```python
from build123d import *

# Parameters (mm, degrees)
SKETCH_1_R               = 4.1
EXTRUDE_1_DEPTH          = 10
SKETCH_2_W               = 10.2
SKETCH_2_H               = 10.2
CUT_EXTRUDE_1_DEPTH      = 5
SKETCH_3_W               = 10
SKETCH_3_H               = 10
EXTRUDE_2_DEPTH          = 10
CUT_EXTRUDE_2_DEPTH      = 64.876521508
CUT_EXTRUDE_2_DEPTH_BACK = 64.876521508
SKETCH_4_R               = 1.6


with BuildPart() as part:
    # ｽｹｯﾁ1 → ﾎﾞｽ - 押し出し1 (new body)
    with BuildSketch(Plane(origin=(0, 0, 0), x_dir=(1, 0, 0), z_dir=(0, 1, 0))):
        with BuildLine():
            Line((-47.110254718, 7.529627927), (-6.738797431, 34.929179684))
            ThreePointArc((-6.738797431, 34.929179684), (5.618470914, 35.603432679), (12, 25))
            Line((12, 25), (12, -25))
            ThreePointArc((12, -25), (5.618470914, -35.603432679), (-6.738797431, -34.929179684))
            Line((-6.738797431, -34.929179684), (-47.110254718, -7.529627927))
            ThreePointArc((-47.110254718, -7.529627927), (-51.1, 0), (-47.110254718, 7.529627927))
        make_face()
        with Locations(Location((-42, 0, 0), (0, 0, 270))):
            Circle(SKETCH_1_R, mode=Mode.SUBTRACT)
    extrude(amount=EXTRUDE_1_DEPTH)

    # ｽｹｯﾁ2 → ｶｯﾄ - 押し出し1 (cut)
    with BuildSketch(Plane.XZ):
        with Locations((0, 25)):
            Rectangle(SKETCH_2_W, SKETCH_2_H)
        with Locations((0, -25)):
            Rectangle(SKETCH_2_W, SKETCH_2_H)
        with Locations((-20, 0)):
            Rectangle(SKETCH_2_W, SKETCH_2_H)
    extrude(amount=-CUT_EXTRUDE_1_DEPTH, mode=Mode.SUBTRACT)

    # ｽｹｯﾁ3 → ﾎﾞｽ - 押し出し2 (add)
    with BuildSketch(Plane(origin=(12, 0, 0), x_dir=(0, 0, -1), z_dir=(1, 0, 0))):
        with Locations((-15, 5)):
            Rectangle(SKETCH_3_W, SKETCH_3_H)
        with Locations((15, 5)):
            Rectangle(SKETCH_3_W, SKETCH_3_H)
    extrude(amount=EXTRUDE_2_DEPTH)

    # ｽｹｯﾁ4 → ｶｯﾄ - 押し出し2 (cut, two sides: drawn at the far end of the back side and taken through both)
    with BuildSketch(Plane.XY.offset(-CUT_EXTRUDE_2_DEPTH_BACK)):
        with Locations((17, 5)):
            Circle(SKETCH_4_R)
    extrude(amount=CUT_EXTRUDE_2_DEPTH + CUT_EXTRUDE_2_DEPTH_BACK, mode=Mode.SUBTRACT)


solid = part.part
```
Input: part model. Units: mm. Frame: model coordinates. A direction names the side the tool comes from. Round coordinates to 2 decimals unless told otherwise and drop trailing zeros. Loops run counter-clockwise (first coordinate to the right, second up) from the corner with the lowest first, then second, coordinate; pieces in that order, holes last. Notation, with made-up numbers: (-22, 86.5) -> (0, 86.5) arc R9 cw to (0, 94.5) -> close; hole circle Ø3 at (-31.5, 46). An arc over 180 degrees is marked (long way). One line per item, written item: value.
(1) Section C-C (y = 1.75). Return the cut outline in (x, z).
Geometry check:
outline: (-47.11, -7.53) -> (-6.74, -34.93) arc R12 ccw to (12, -25) -> (12, -20) -> (22, -20) -> (22, -10) -> (12, -10) -> (12, 10) -> (22, 10) -> (22, 20) -> (12, 20) -> (12, 25) arc R12 ccw to (-6.74, 34.93) -> (-47.11, 7.53) arc R9.1 ccw to start; hole circle Ø8.2 at (-42, 0); hole (-25.1, -5.1) -> (-14.9, -5.1) -> (-14.9, 5.1) -> (-25.1, 5.1) -> close; hole (-5.1, -30.1) -> (5.1, -30.1) -> (5.1, -19.9) -> (-5.1, -19.9) -> close; hole (-5.1, 19.9) -> (5.1, 19.9) -> (5.1, 30.1) -> (-5.1, 30.1) -> close
(2) Set-up query: faces 5 (the face through (0, 5, 25)), 6 (the face through (15, 5, 10)), 7 (the face through (15, 5, 20)), 8 (the face through (22, 5, 15)). Return all of +Z, -Z, +X, -X, +Y, -Y with unobstructed straight access to the full face (end or side cutting, diameter ignored); none if empty.
Geometry check:
face 5: -Y
face 6: +X, +Y, -Y
face 7: +Z, +X, +Y, -Y
face 8: +Z, -Z, +X, +Y, -Y
(3) Material intervals for line 1 (Y direction, x = 17, z = -12.25); line 2 (Z direction, x = 17, y = 2.25); line 3 (X direction, y = 8, z = 0), sorted ascending. Write a range as [from, to].
Geometry check:
line 1: [0, 3.4], [6.6, 10]
line 2: [-20, -10], [10, 20]
line 3: [-51.1, -46.1], [-37.9, 12]
(4) Pin query (flat end, axial travel): pin 1 (2 mm diameter, centred on y = 5, z = 13, fed in from -X); pin 2 (3 mm diameter, centred on x = 17, y = 5, fed in from +Z); pin 3 (6 mm diameter, centred on x = 1, y = 1.5, fed in from -Z); pin 4 (4 mm diameter, centred on x = 17, y = 5, fed in from +Z). Return the tip coordinate at first contact, or that it passes through.
Geometry check:
pin 1: x = -40.52
pin 2: through
pin 3: z = -37
pin 4: z = 20
(5) Mould query, pull axis Z, two halves, no side actions, for faces 1 (the face through (-51.1, 4.9, 0.1)), 2 (the face through (-20, 2, -5.1)), 3 (the face through (5.779, 4.93, 35.517)), 4 (the face through (15.4, 5.07, 14.93)). Classes: pulls with the +Z half, pulls with the -Z half, needs draft (parallel to the pull), parting line crosses it, or undercut.
Geometry check:
face 1: parting line crosses it
face 2: undercut
face 3: pulls with the +Z half
face 4: needs draft
(6) Section A-A (z = 0). Return the cut outline in (x, y).
Geometry check:
outline: (-51.1, 0) -> (-46.1, 0) -> (-46.1, 10) -> (-51.1, 10) -> close; (-37.9, 0) -> (-25.1, 0) -> (-25.1, 5) -> (-14.9, 5) -> (-14.9, 0) -> (12, 0) -> (12, 10) -> (-37.9, 10) -> close
(7) Section D-D (x = -41). Return the cut outline in (y, z), plus the area to 3 significant figures.
Geometry check:
outline: (0, -11.68) -> (10, -11.68) -> (10, -3.98) -> (0, -3.98) -> close; (0, 3.98) -> (10, 3.98) -> (10, 11.68) -> (0, 11.68) -> close
area: 154 mm2
(8) Section B-B (x = 17). Return the cut outline in (y, z).
Geometry check:
outline: (0, -20) -> (3.4, -20) -> (3.4, -10) -> (0, -10) -> close; (0, 10) -> (3.4, 10) -> (3.4, 20) -> (0, 20) -> close; (6.6, -20) -> (10, -20) -> (10, -10) -> (6.6, -10) -> close; (6.6, 10) -> (10, 10) -> (10, 20) -> (6.6, 20) -> close
